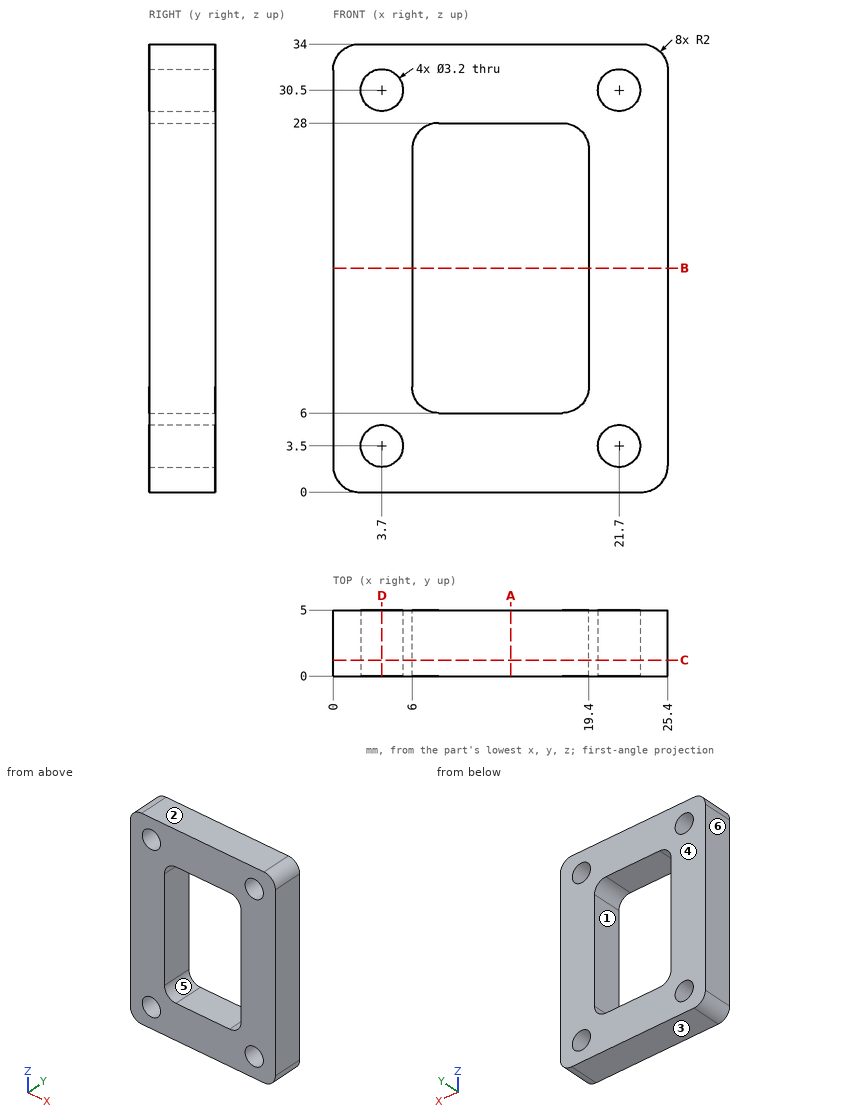
Source: three-view drawing plus pictorial views. Frame: mm from the lowest corner of the part. A direction names the side the tool comes from. Round coordinates to 2 decimals unless told otherwise and drop trailing zeros. Loops run counter-clockwise (first coordinate to the right, second up) from the corner with the lowest first, then second, coordinate; pieces in that order, holes last.
Q1. Section A-A on x = 13.5. Return loops of the section in (y, z).
Q2. Section D-D on x = 3.7. Return loops of the section in (y, z).
Q3. Pull-direction query (Z, two-part tool) for the marked faces 1, 2, 3 and 4; classes: released by +Z, released by -Z, zero draft, split by the parting line, or undercut.
Q4. Section C-C on y = 1.2. Return loops of the section in (x, z).
Q5. Material intervals for L1, parallel to X at y = 1.35, z = 30.5; L2, parallel to Z at x = 9.5, y = 3.05; L3, parallel to X at y = 3.1, z = 13.5, sorted ascending.
Q6. Section B-B on z = 17. Return loops of the section in (x, y).
Q7. Access query for the marked faces 5 and 6. Directions: +Z, -Z, +X, -X, +Y, -Y. A direction counts if a zero-diameter tool reaches every point of the face in a straight line with its end or side. Return the directions, or none.
Evaluation:
1. outline: (0, 0) - (5, 0) - (5, 6) - (0, 6) - close; (0, 28) - (5, 28) - (5, 34) - (0, 34) - close
2. outline: (0, 0) - (5, 0) - (5, 1.9) - (0, 1.9) - close; (0, 5.1) - (5, 5.1) - (5, 28.9) - (0, 28.9) - close; (0, 32.1) - (5, 32.1) - (5, 34) - (0, 34) - close
3. face 1: undercut
3. face 2: released by +Z
3. face 3: released by -Z
3. face 4: zero draft
4. outline: (0, 2) arc R2 ccw to (2, 0) - (23.4, 0) arc R2 ccw to (25.4, 2) - (25.4, 32) arc R2 ccw to (23.4, 34) - (2, 34) arc R2 ccw to (0, 32) - close; hole circle Ø3.2 at (3.7, 3.5); hole circle Ø3.2 at (3.7, 30.5); hole (6, 8) arc R2 ccw to (8, 6) - (17.4, 6) arc R2 ccw to (19.4, 8) - (19.4, 26) arc R2 ccw to (17.4, 28) - (8, 28) arc R2 ccw to (6, 26) - close; hole circle Ø3.2 at (21.7, 3.5); hole circle Ø3.2 at (21.7, 30.5)
5. L1: x = 0 to 2.1, 5.3 to 20.1, 23.3 to 25.4
5. L2: z = 0 to 6, 28 to 34
5. L3: x = 0 to 6, 19.4 to 25.4
6. outline: (0, 0) - (6, 0) - (6, 5) - (0, 5) - close; (19.4, 0) - (25.4, 0) - (25.4, 5) - (19.4, 5) - close
7. face 5: +Y, -Y
7. face 6: +Z, -Z, -X, +Y, -Y
